Work out the finished part from the listing and answer in its coordinate system (mm). Face numbers are marked on the shaded views. A direction names the side the tool comes from. Coordinates: 2 decimals unless noted, no trailing zeros. Loops run counter-clockwise (first coordinate to the right, second up) from the corner with the lowest first, then second, coordinate; pieces in that order, holes last. Notation, with made-up numbers: M 28,26.25 L 48,26.25 A20 cw 48,39.25 Z; hole C -8.75,35 d2. An arc over 180 degrees is marked long. Write each question's results on one line, items separated by ' | '.
```python
from build123d import *

# Parameters (mm, degrees)
EXTRUDE_1_DEPTH                = 6
HOLE_WIZARD_M1_6_1_D           = 1.25
HOLE_WIZARD_M1_6_1_CSINK_D     = 1.65
HOLE_WIZARD_M1_6_1_CSINK_ANGLE = 90


with BuildPart() as part:
    # 草图2 → 凸台-拉伸1 (new body)
    with BuildSketch(Plane(origin=(0, 0, 0), x_dir=(1, 0, 0), z_dir=(0, 1, 0))):
        with BuildLine():
            Line((3.07408523, 0.4), (6.07408523, 0.4))
            Line((6.07408523, 0.4), (6.07408523, 0.6))
            Line((6.07408523, 0.6), (3.244996148, 0.6))
            ThreePointArc((3.244996148, 0.6), (-3.3, 0), (3.244996148, -0.6))
            Line((3.244996148, -0.6), (6.07408523, -0.6))
            Line((6.07408523, -0.6), (6.07408523, -0.4))
            Line((6.07408523, -0.4), (3.07408523, -0.4))
            ThreePointArc((3.07408523, -0.4), (-3.1, 0), (3.07408523, 0.4))
        make_face()
    extrude(amount=EXTRUDE_1_DEPTH)

    # M1.6 螺纹孔1 (through all)
    with Locations(Plane(origin=(0, 0, -0.6), x_dir=(-1, 0, 0), z_dir=(0, 0, -1))):
        with Locations((-4.57408523, 4.8), (-4.57408523, 1.2)):
            CounterSinkHole(HOLE_WIZARD_M1_6_1_D / 2, HOLE_WIZARD_M1_6_1_CSINK_D / 2, counter_sink_angle=HOLE_WIZARD_M1_6_1_CSINK_ANGLE)


solid = part.part
```
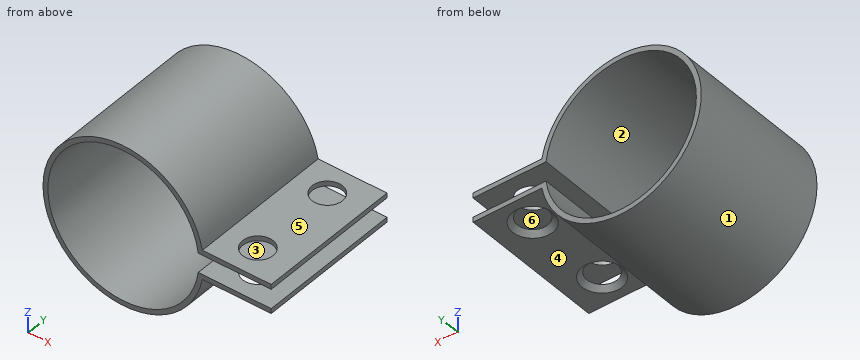
1) Given pin 1 Ø2 at (y, z) = (2.5, 1) entering from -X; pin 2 Ø3 at (x, y) = (4, 3.5) entering from +Z; pin 3 Ø2.5 at (x, y) = (5, 3) entering from +Z; pin 4 Ø1.4 at (x, y) = (5, 2.5) entering from -Z, each flat-ended and moving along its own axis, determine where each tip first touches the part or whether it passes through.
Check result:
pin 1: x = -3.3 | pin 2: z = 2.15 | pin 3: z = 0.6 | pin 4: z = -0.6
2) Find section C-C, the plane z = -2. Give the vertices of the cut face in (x, y), and give its area (3 significant figures).
Check result:
outline: M -2.62,0 L -2.37,0 L -2.37,6 L -2.62,6 Z; M 2.37,0 L 2.62,0 L 2.62,6 L 2.37,6 Z | area: 3.08 mm^2
3) Which of the six approach directions +Z, -Z, +X, -X, +Y, -Y give full straight-line access (tool end or side, diameter ignored) to the marked faces 4, 5 and 6?
Check result:
face 4: -Z, +X, +Y, -Y | face 5: +Z, +X, +Y, -Y | face 6: +X, +Y, -Y
4) Find section D-D, the plane z = 0. Give the vertices of the cut face in (x, y).
Check result:
outline: M -3.3,0 L -3.1,0 L -3.1,6 L -3.3,6 Z
5) Find section A-A, the plane x = 0. Give the vertices of the cut face in (y, z).
Check result:
outline: M 0,-3.3 L 6,-3.3 L 6,-3.1 L 0,-3.1 Z; M 0,3.1 L 6,3.1 L 6,3.3 L 0,3.3 Z
6) Straight lines are drawn through the part: probe 1 along X at (y, z) = (1.35, 0.5); probe 2 along Z at (x, y) = (5, 2); probe 3 along Z at (x, y) = (0, 0.55). For each, find the intervals that lie inside material, in ascending order. Write a range as [from, to].
Check result:
probe 1: [-3.26, -3.06], [3.06, 3.97], [5.18, 6.07] | probe 2: [-0.6, -0.4], [0.4, 0.6] | probe 3: [-3.3, -3.1], [3.1, 3.3]
7) For a pull along X with two mould halves and no side action, classify the marked faces 1, 2 and 3 as released by +X, released by -X, zero draft, split by the parting line, or undercut.
Check result:
face 1: split by the parting line | face 2: undercut | face 3: zero draft
8) Find section B-B, the plane y = 4.8. Give the vertices of the cut face in (x, z) (3 decimals).
Check result:
outline: M 3.074,-0.4 A3.1 cw long 3.074,0.4 L 3.949,0.4 L 3.949,0.6 L 3.245,0.6 A3.3 ccw long 3.245,-0.6 L 3.749,-0.6 L 3.949,-0.4 Z; M 5.199,-0.4 L 5.399,-0.6 L 6.074,-0.6 L 6.074,-0.4 Z; M 5.199,0.4 L 6.074,0.4 L 6.074,0.6 L 5.199,0.6 Z
